Check sheet for the drawn part. Datum: minimum x, y, z corner. Units: mm. A direction names the side the tool comes from. Coordinates: 2 decimals unless noted, no trailing zeros. Write each loop counter-clockwise with the first axis right and the second up, starting at its lowest first coordinate (ties: lowest second). Pieces come first, ordered by that corner, then holes. Notation, with made-up numbers: (42, -15.75) -> (90, -15.75) arc R16 cw to (90, 4.25) -> close; hole circle Ø5 at (42.5, 26). An arc over 180 degrees is marked (long way). Write item = value, one per line. Start each with the question number.
(1) Mould release check, pull along X, two halves, no side actions. Record for the marked faces 1, 2 and 3: released by +X, released by -X, zero draft, split by the parting line, or undercut.
(2) Section check B-B (y = 31). Record the cut outline in (x, z) (1 decimal).
(3) Gauge pin test, flat ends, axial feed: pin 1 Ø4 at (y, z) = (27.83, 4.43) entering from -X; pin 2 Ø4 at (x, z) = (6, 6.5) entering from -Y. Record the tip position at first contact, or that the pin passes through.
(4) Section check A-A (z = 2.75). Record the cut outline in (x, y) (1 decimal).
(5) Material ranges on probe 1 along X at (y, z) = (33, 1.5) (1 decimal); probe 2 along Z at (x, y) = (9.5, 10); probe 3 along Z at (x, y) = (8.5, 41), recorded low to high. Write a range as [from, to].
(6) Section check D-D (z = 5.5). Record the cut outline in (x, y) (1 decimal), plus the area to 3 significant figures.
(7) Set-up check for the marked faces 4 and 5: record each of +Z, -Z, +X, -X, +Y, -Y from which the full face is reachable in a straight line by a thin tool's end or side.
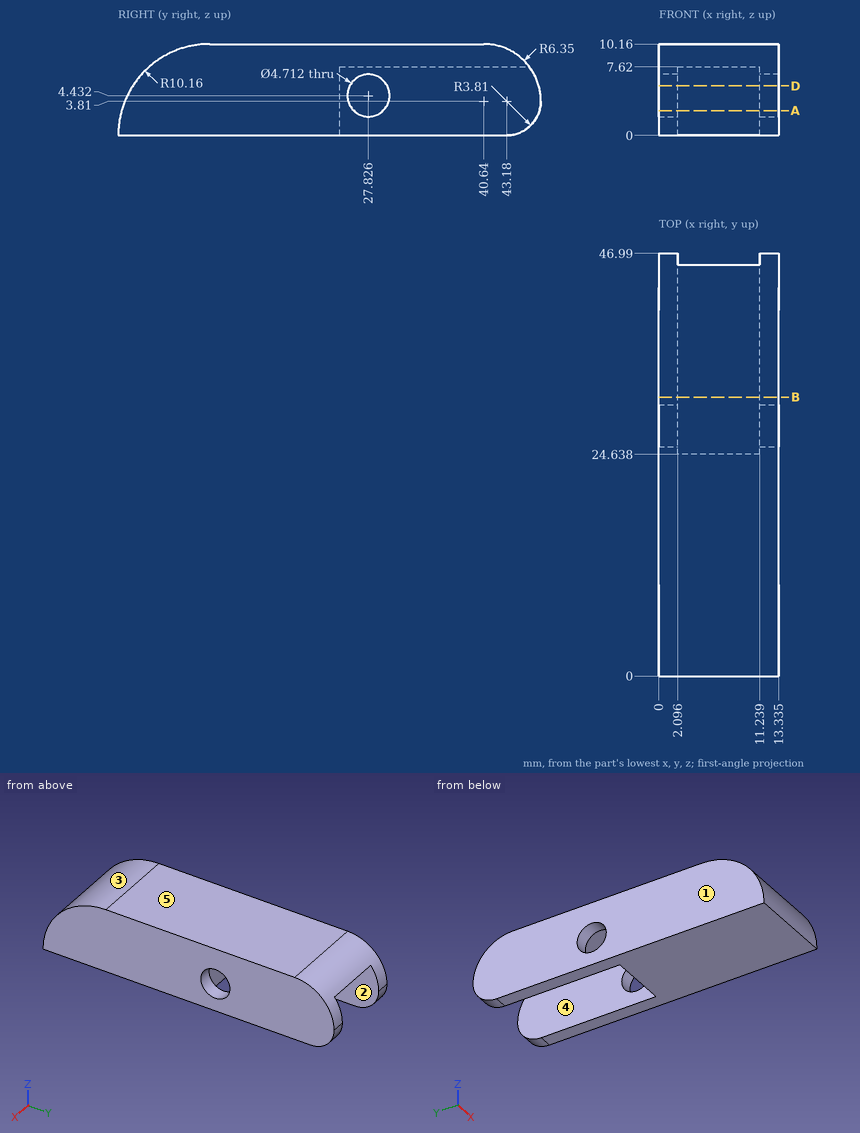
Response:
q1.face_1 = released by -X
q1.face_2 = undercut
q1.face_3 = zero draft
q2.outline = (0, 0) -> (2.1, 0) -> (2.1, 7.6) -> (11.2, 7.6) -> (11.2, 0) -> (13.3, 0) -> (13.3, 10.2) -> (0, 10.2) -> close
q3.pin_1 = through
q3.pin_2 = 1.05
q4.outline = (0, 0.4) -> (13.3, 0.4) -> (13.3, 26.2) -> (11.2, 26.2) -> (11.2, 24.6) -> (2.1, 24.6) -> (2.1, 26.2) -> (0, 26.2) -> close; (0, 29.5) -> (2.1, 29.5) -> (2.1, 46.8) -> (0, 46.8) -> close; (11.2, 29.5) -> (13.3, 29.5) -> (13.3, 46.8) -> (11.2, 46.8) -> close
q5.probe_1 = [0, 2.1], [11.2, 13.3]
q5.probe_2 = [0, 10.16]
q5.probe_3 = [7.62, 10.15]
q6.outline = (0, 1.6) -> (13.3, 1.6) -> (13.3, 25.7) -> (11.2, 25.7) -> (11.2, 24.6) -> (2.1, 24.6) -> (2.1, 25.7) -> (0, 25.7) -> close; (0, 29.9) -> (2.1, 29.9) -> (2.1, 46.8) -> (0, 46.8) -> close; (11.2, 29.9) -> (13.3, 29.9) -> (13.3, 46.8) -> (11.2, 46.8) -> close
q6.area = 382 mm2
q7.face_4 = -Z, +Y
q7.face_5 = +Z, +X, -X, +Y, -Y
